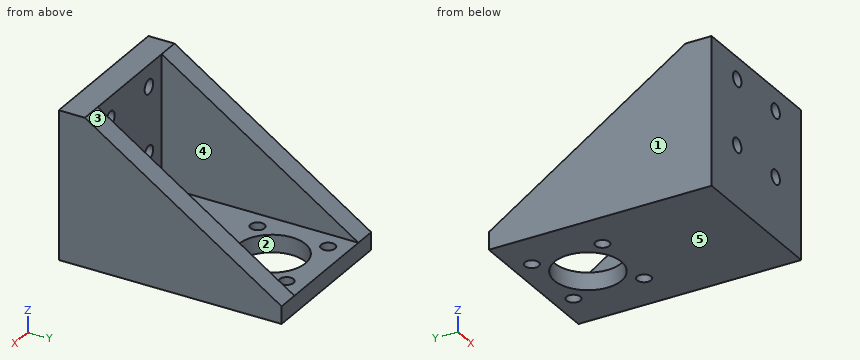
Autodesk Inventor part; units mm, degrees
ref_plane "YZ Plane" through (0, 0, 0) normal (1, 0, 0) x (0, 1, 0)
ref_plane "XZ Plane" through (0, 0, 0) normal (0, 1, 0) x (-1, 0, 0)
ref_plane "XY Plane" through (0, 0, 0) normal (0, 0, 1) x (1, 0, 0)
sketch "Sketch1" plane through (0, 0, 0) normal (0, 0, 1) x (1, 0, 0)
  line L0 (-35, -25) -> (35, -25)
  line L1 (35, -25) -> (35, 25)
  line L2 (35, 25) -> (-35, 25)
  line L3 (-35, 25) -> (-35, -25)
  line L4 (-35, -25) -> (35, 25) construction
  line L5 (35, -25) -> (-35, 25) construction
  circle A0 centre (0, 0) radius 15.4
  dimension "d0" = 70
  dimension "d1" = 50
  dimension "d2" = 30.8
extrude "Extrusion1" add sketch "Sketch1" along normal blind 8
sketch "Sketch2" plane through (0, 0, 8) normal (0, 0, 1) x (1, 0, 0)
  line L0 (35, -25) -> (35, 25)
  line L1 (35, 25) -> (-35, 25)
  line L2 (-35, 25) -> (-35, -25)
  line L3 (-35, -25) -> (35, -25)
  circle A0 centre (0, 0) radius 15.4
  line L4 (16.25, -16.25) -> (-16.25, -16.25) construction
  line L5 (-16.25, -16.25) -> (-16.25, 16.25) construction
  line L6 (-16.25, 16.25) -> (16.25, 16.25) construction
  line L7 (16.25, 16.25) -> (16.25, -16.25) construction
  line L8 (16.25, -16.25) -> (-16.25, 16.25) construction
  line L9 (-16.25, -16.25) -> (16.25, 16.25) construction
  dimension "d5" = 32.5
  dimension "d6" = 32.5
hole "Hole1" at (-16.25, 16.25, 8) at (16.25, 16.25, 8) at (16.25, -16.25, 8) at (-16.25, -16.25, 8) direction (0, 0, -1) diameter 6.4 end through all
sketch "Sketch3" plane through (0, 0, 8) normal (0, 0, 1) x (1, 0, 0)
  circle A0 centre (0, 0) radius 15.4
  circle A1 centre (-16.25, -16.25) radius 3.2
  circle A2 centre (16.25, -16.25) radius 3.2
  circle A3 centre (16.25, 16.25) radius 3.2
  circle A4 centre (-16.25, 16.25) radius 3.2
  line L0 (35, -25) -> (35, 25)
  line L1 (35, 25) -> (-35, 25)
  line L2 (-35, 25) -> (-35, -25)
  line L3 (-35, -25) -> (35, -25)
  circle A5 centre (0, 0) radius 15.4
  line L4 (-35, -25) -> (35, -25)
  line L5 (35, -25) -> (35, -77.5)
  line L6 (35, -77.5) -> (-35, -77.5)
  line L7 (-35, -77.5) -> (-35, -25)
  dimension "d14" = 77.5
extrude "Extrusion2" add sketch "Sketch3" against normal up to surface (8 mm away) contours L5 L6 L7 L3
sketch "Sketch4" plane through (-35, 25, 0) normal (-1, 0, 0) x (0, 0, 1)
  line L0 (0, 0) -> (0, -102.5)
  line L1 (8, -102.5) -> (0, -102.5)
  line L2 (8, 0) -> (8, -102.5)
  line L3 (0, 0) -> (8, 0)
  line L4 (8, -102.5) -> (68, -102.5)
  line L5 (68, -102.5) -> (68, -90.5)
  line L6 (68, -90.5) -> (8, -90.5)
  line L7 (8, -90.5) -> (8, -102.5)
  line L8 (68, -90.5) -> (8, 0)
  point P0 (0, -25)
  dimension "d17" = 60
  dimension "d18" = 12
extrude "Extrusion3" add sketch "Sketch4" against normal blind 10 contours L8 L6 L2 | L2 L6 L5 L4
mirror "Mirror1" about plane through (0, 0, 0) normal (1, 0, 0) of "Extrusion3"
sketch "Sketch5" plane through (-35, -77.5, 0) normal (0, -1, 0) x (1, 0, 0)
  line L0 (10, 68) -> (10, 8)
  line L1 (60, 68) -> (60, 8)
  line L2 (10, 8) -> (60, 8)
  line L3 (10, 68) -> (60, 68)
  point P0 (35, 0)
extrude "Extrusion4" add sketch "Sketch5" against normal blind 12
sketch "Sketch6" plane through (-35, -65.5, 0) normal (0, 1, 0) x (1, 0, 0)
  line L0 (10, -68) -> (10, -8)
  line L1 (10, -68) -> (60, -68)
  line L2 (60, -8) -> (60, -68)
  line L3 (10, -8) -> (60, -8)
  line L4 (50, -18) -> (50, -58) construction
  line L5 (50, -58) -> (20, -58) construction
  line L6 (20, -58) -> (20, -18) construction
  line L7 (20, -18) -> (50, -18) construction
  point P0 (35, 0)
  dimension "d23" = 10
hole "Hole2" at (-15, -65.5, 18) at (-15, -65.5, 58) at (15, -65.5, 18) at (15, -65.5, 58) direction (0, -1, 0) diameter 6.6 end through all
move faces "Move1" translate (0, 0, 10) faces at (15.2655, -69.5, 21.2893) (-14.7345, -69.5, 21.2893)
properties part number "Part6_3DPrint"
Geometry check sheet. Reference: the model listing, model coordinates, mm. Face numbers are marked on the shaded views. A direction names the side the tool comes from. Give positions to 0.01 mm unless a question says otherwise; leave off trailing zeros. Write each loop counter-clockwise with the first axis right and the second up, starting at its lowest first coordinate (ties: lowest second). Pieces come first, ordered by that corner, then holes. Notation, with made-up numbers: (15, 65) - (38, 65) arc R24 cw to (38, 80) - close; hole circle Ø10 at (12, 16). An arc over 180 degrees is marked (long way). Put each result on its own line as item: value.
1. Thickness scan on line 1 (Y direction, x = 16, z = 5); line 2 (X direction, y = -71.5, z = 58); line 3 (Z direction, x = 15, y = -73.75). Record the ranges inside material, lowest first.
Ans:
line 1: y = -77.5 to -19.44, -13.06 to 13.06, 19.44 to 25
line 2: x = -35 to -18.3, -11.7 to 11.7, 18.3 to 35
line 3: z = 0 to 24.7, 31.3 to 54.7, 61.3 to 68
2. Sectioned sample at A-A, the plane x = 0. Enter the section's corners in (y, z), plus the area to 3 significant figures.
Ans:
outline: (-77.5, 0) - (-15.4, 0) - (-15.4, 8) - (-65.5, 8) - (-65.5, 68) - (-77.5, 68) - close; (15.4, 0) - (25, 0) - (25, 8) - (15.4, 8) - close
area: 1,290 mm²
3. Go/stop test with flat-tipped pins: pin 1 (2 mm diameter, centred on x = 12, y = -40, fed in from -Z); pin 2 (25 mm diameter, centred on x = 12, y = -20.5, fed in from +Z); pin 3 (10 mm diameter, centred on x = 2.5, z = 50.5, fed in from +Y). Record where each tip stops, or that it passes through.
Ans:
pin 1: stops at z = 0
pin 2: stops at z = 8
pin 3: stops at y = -65.5
4. Sectioned sample at C-C, the plane z = 58. Enter the section's corners in (x, y).
Ans:
outline: (-35, -77.5) - (-18.3, -77.5) - (-18.3, -65.5) - (-25, -65.5) - (-25, -50.42) - (-35, -50.42) - close; (-11.7, -77.5) - (11.7, -77.5) - (11.7, -65.5) - (-11.7, -65.5) - close; (18.3, -77.5) - (35, -77.5) - (35, -50.42) - (25, -50.42) - (25, -65.5) - (18.3, -65.5) - close
5. Sectioned sample at B-B, the plane y = 0. Enter the section's corners in (x, z).
Ans:
outline: (-35, 0) - (-15.4, 0) - (-15.4, 8) - (-25, 8) - (-25, 24.57) - (-35, 24.57) - close; (15.4, 0) - (35, 0) - (35, 24.57) - (25, 24.57) - (25, 8) - (15.4, 8) - close
6. Set-up check for the marked faces 4 and 5: record each of +Z, -Z, +X, -X, +Y, -Y from which the full face is reachable in a straight line by a thin tool's end or side.
Ans:
face 4: +Z, +Y
face 5: -Z, +X, -X, +Y, -Y
7. Draft check along Y on the marked faces 1, 2 and 3. Enter one of: +Y half, -Y half, draft (parallel to the pull), parting line (faces both ways), or undercut.
Ans:
face 1: draft
face 2: undercut
face 3: +Y half
8. Sectioned sample at D-D, the plane y = -51.5. Enter the section's corners in (x, z), plus the area to 3 significant figures.
Ans:
outline: (-35, 0) - (35, 0) - (35, 58.72) - (25, 58.72) - (25, 8) - (-25, 8) - (-25, 58.72) - (-35, 58.72) - close
area: 1,570 mm²
